from build123d import *

# Parameters (mm, degrees)
SKETCH1_W                   = 20
SKETCH1_H                   = 16
BOSS_EXTRUDE1_DEPTH         = 11.5
CUT_EXTRUDE1_DEPTH          = 23.096379794
M3_TAPPED_HOLE1_D           = 2.5
M3_TAPPED_HOLE1_DEPTH       = 3.5
M3_TAPPED_HOLE1_CBORE_D     = 3
M3_TAPPED_HOLE1_CBORE_DEPTH = 3
M3_TAPPED_HOLE1_TIP         = 0.751075774
HOLE1_D                     = 1.5
HOLE1_DEPTH                 = 4.5
HOLE1_CBORE_D               = 2
HOLE1_CBORE_DEPTH           = 2
M6_TAPPED_HOLE1_D           = 6
M3_TAPPED_HOLE2_D           = 3
CHAMFER1_SIZE               = 0.5


with BuildPart() as part:
    # Sketch1 → Boss-Extrude1 (new body)
    with BuildSketch(Plane(origin=(0, 0, 0), x_dir=(1, 0, 0), z_dir=(0, 1, 0))):
        Rectangle(SKETCH1_W, SKETCH1_H)
    extrude(amount=BOSS_EXTRUDE1_DEPTH)

    # Sketch2 → Cut-Extrude1 (cut, through all)
    with BuildSketch(Plane.XY.offset(8)):
        with BuildLine():
            Line((-4.40473751, 4.75), (-10, 4.75))
            Line((-10, 4.75), (-10, 4))
            Line((-10, 4), (-10, 3.25))
            Line((-10, 3.25), (-4.40473751, 3.25))
            ThreePointArc((-4.40473751, 3.25), (1.5, 4), (-4.40473751, 4.75))
        make_face()
    extrude(amount=-CUT_EXTRUDE1_DEPTH, mode=Mode.SUBTRACT)

    # M3 Tapped Hole1
    with Locations(Plane.XY.offset(8)):
        with Locations((6.5, 4.8)):
            CounterBoreHole(M3_TAPPED_HOLE1_D / 2, M3_TAPPED_HOLE1_CBORE_D / 2, M3_TAPPED_HOLE1_CBORE_DEPTH, depth=M3_TAPPED_HOLE1_DEPTH)
            with Locations((0, 0, -(M3_TAPPED_HOLE1_DEPTH + M3_TAPPED_HOLE1_TIP / 2))):  # 118° drill point
                Cone(0, M3_TAPPED_HOLE1_D / 2, M3_TAPPED_HOLE1_TIP, mode=Mode.SUBTRACT)

    # Hole1
    with Locations(Plane.XY.offset(8)):
        with Locations((8, 2)):
            CounterBoreHole(HOLE1_D / 2, HOLE1_CBORE_D / 2, HOLE1_CBORE_DEPTH, depth=HOLE1_DEPTH)

    # M6 Tapped Hole1 (through all)
    with Locations(Plane(origin=(0, 11.5, 0), x_dir=(1, 0, 0), z_dir=(0, 1, 0))):
        with Locations((5.5, 0)):
            Hole(M6_TAPPED_HOLE1_D / 2)

    # M3 Tapped Hole2 (through all)
    with Locations(Plane(origin=(0, 11.5, 0), x_dir=(1, 0, 0), z_dir=(0, 1, 0))):
        with Locations((-7.5, 0)):
            Hole(M3_TAPPED_HOLE2_D / 2)

    # Chamfer1
    chamfer1_edges = [part.edges().sort_by_distance(p)[0] for p in [
        (-10, 11.5, 0),
        (0, 11.5, 8),
        (-10, 1.625, 8),
        (-10, 1.625, -8),
        (10, 11.5, 0),
        (0, 0, 8),
        (-10, 0, 0),
        (0, 0, -8),
        (10, 0, 0),
        (0, 11.5, -8),
        (10, 5.75, 8),
        (-10, 8.125, 8),
        (-10, 8.125, -8),
        (10, 5.75, -8),
    ]]
    chamfer(chamfer1_edges, length=CHAMFER1_SIZE)


solid = part.part
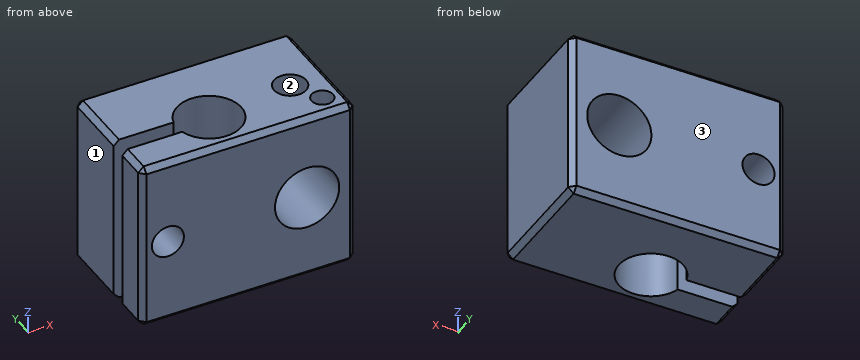
Input: part model. Units: mm. Frame: model coordinates. Face numbers are marked on the shaded views. Give positions to 0.01 mm unless a question says otherwise; leave off trailing zeros. Loops run counter-clockwise (first coordinate to the right, second up) from the corner with the lowest first, then second, coordinate; pieces in that order, holes last. Notation, with made-up numbers: M 3.5,57 L 34.5,57 A21 ccw 34.5,89 Z; hole C 66.25,6.25 d3. An arc over 180 degrees is marked long. Use one line per item in the form item = value.
1. Section query B-B, the plane y = 6.75. Return the cut outline in (x, z).
Numbers:
outline = M -10,-7.5 L -9.5,-8 L -2.7,-8 L -2.7,8 L -9.5,8 L -10,7.5 Z; M -0.3,-8 L 9.5,-8 L 10,-7.5 L 10,7.5 L 9.5,8 L -0.3,8 Z; hole C -7.5,0 d3; hole C 5.5,0 d6
2. First-contact query: pin 1 (4.5 mm diameter, centred on x = -8.5, z = 0, fed in from -Y); pin 2 (0.9 mm diameter, centred on x = 7, y = 4.5, fed in from +Z); pin 3 (1.6 mm diameter, centred on x = 8, y = 2, fed in from +Z). Flat tips, straight axial feed; report the tip coordinate or a pass-through.
Numbers:
pin_1 = 0
pin_2 = 4.37
pin_3 = 6
3. Section query C-C, the plane z = 6.25. Return the cut outline in (x, y).
Numbers:
outline = M -10,0.5 L -9.5,0 L 9.5,0 L 10,0.5 L 10,11 L 9.5,11.5 L -9.5,11.5 L -10,11 L -10,4.75 L -4.4,4.75 A3 cw long -4.4,3.25 L -10,3.25 Z; hole C 6.5,4.8 d3; hole C 8,2 d2
4. Section query D-D, the plane x = -1.5. Return the cut outline in (y, z), and give its area (3 significant figures).
Numbers:
outline = M 0,-7.5 L 0.5,-8 L 1,-8 L 1,8 L 0.5,8 L 0,7.5 Z; M 7,-8 L 11,-8 L 11.5,-7.5 L 11.5,7.5 L 11,8 L 7,8 Z
area = 87.5 mm²
5. Pull-direction query (X, two-part tool) for the marked faces 1, 2 and 3; classes: released by +X, released by -X, zero draft, split by the parting line, or undercut.
Numbers:
face_1 = released by -X
face_2 = undercut
face_3 = zero draft
6. Section query A-A, the plane z = 0. Return the cut outline in (x, y), and give its area (3 significant figures).
Numbers:
outline = M -10,0.5 L -9.5,0 L -9,0 L -9,3.25 L -10,3.25 Z; M -10,4.75 L -9,4.75 L -9,11.5 L -9.5,11.5 L -10,11 Z; M -6,0 L 2.5,0 L 2.5,11.5 L -6,11.5 L -6,4.75 L -4.4,4.75 A3 cw long -4.4,3.25 L -6,3.25 Z; M 8.5,0 L 9.5,0 L 10,0.5 L 10,11 L 9.5,11.5 L 8.5,11.5 Z
area = 93.9 mm²
7. Line query: L1, parallel to Z at x = 5.5, y = 2.5; L2, parallel to Y at x = -6.25, z = 6.5; L3, parallel to Z at x = -7.5, y = 8. Output: solid intervals per line, ascending.
Numbers:
L1 = -8 to -3, 3 to 8
L2 = 0 to 3.25, 4.75 to 11.5
L3 = -8 to -1.5, 1.5 to 8
